Input: part model. Units: mm. Frame: model coordinates. Give positions to 0.01 mm unless a question says otherwise; leave off trailing zeros. Write each loop counter-clockwise with the first axis right and the second up, starting at its lowest first coordinate (ties: lowest second). Pieces come first, ordered by that corner, then holes. Notation, with made-up numbers: (-19, 47) - (-9, 47) arc R19 ccw to (-9, 73) - close; hole circle Ø11 at (-31.5, 76.25). An arc over 180 degrees is marked (long way). Answer as a JSON object with one key per item and string values. Group by question number.
from build123d import *

# Parameters (mm, degrees)
F0_W     = 15
F0_H     = 3.2
F1_DEPTH = 3.2


with BuildPart() as f1:
    # F0 (on Top) → F1 (new body)
    with BuildSketch(Plane.XY):
        Polygon((28.25105, 0), (33.25105, 0), (33.25105, 43.6), (28.25105, 43.6), (13.25105, 43.6), (-6.74895, 43.6), (-21.74895, 43.6), (-46.44895, 43.6), (-46.44895, 0), (-21.74895, 0), (-6.74895, 0), (13.25105, 0), align=None)
        with Locations((20.75105, -1.6)):
            Rectangle(F0_W, F0_H)
        with Locations((20.75105, 45.2)):
            Rectangle(F0_W, F0_H)
        with Locations((-14.24895, -1.6)):
            Rectangle(F0_W, F0_H)
        with Locations((-14.24895, 45.2)):
            Rectangle(F0_W, F0_H)
    extrude(amount=F1_DEPTH)


solid = f1.part
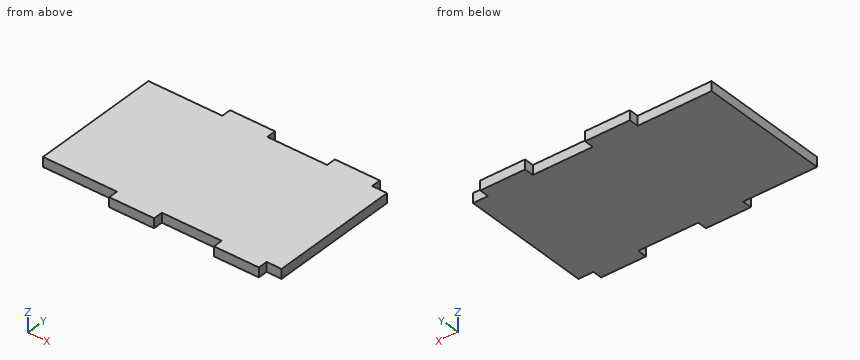
1) Cut plane A-A on z = 1.3. Return the cut outline in (x, y), and give its area (3 significant figures).
2) Line query: line 1 along X through (y, z) = (44.5, 0.95); line 2 along Y through (x, z) = (30.5, 0.4). Output: solid intervals per line, ascending. Write a range as from..to.
3) Pin query (flat end, axial travel): P1, Ø1.6, axis at y = 45, z = 2, coming from the -X side; P2, Ø1.6, axis at x = 30, z = 1, coming from the -Y side; P3, Ø1, axis at x = 30, z = 1, coming from the +Y side. Return the tip coordinate at first contact, or that it passes through.
4) Cut plane B-B on x = -37.5. Return the cut outline in (y, z).
Filled in:
{
 "1": {"outline": "(-46.45, 0) - (-21.75, 0) - (-21.75, -3.2) - (-6.75, -3.2) - (-6.75, 0) - (13.25, 0) - (13.25, -3.2) - (28.25, -3.2) - (28.25, 0) - (33.25, 0) - (33.25, 43.6) - (28.25, 43.6) - (28.25, 46.8) - (13.25, 46.8) - (13.25, 43.6) - (-6.75, 43.6) - (-6.75, 46.8) - (-21.75, 46.8) - (-21.75, 43.6) - (-46.45, 43.6) - close", "area": "3,670 mm²"},
 "2": {"line 1": "x = -21.75..-6.75, 13.25..28.25", "line 2": "y = 0..43.6"},
 "3": {"P1": "stops at x = -21.75", "P2": "stops at y = 0", "P3": "stops at y = 43.6"},
 "4": {"outline": "(0, 0) - (43.6, 0) - (43.6, 3.2) - (0, 3.2) - close"}
}
